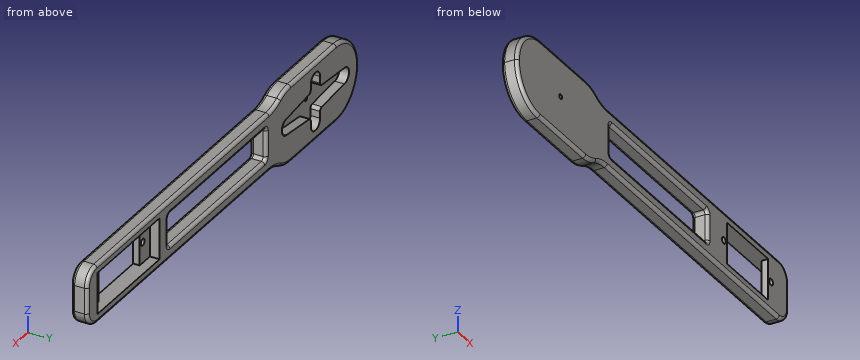
```python
from build123d import *

# Parameters (mm, degrees)
BOSS_EXTRUDE1_DEPTH = 6
CUT_EXTRUDE2_START  = -1
CUT_EXTRUDE2_DEPTH  = 1
SKETCH17_R          = 0.75
CUT_EXTRUDE8_DEPTH  = 4
SKETCH18_R          = 0.75
CUT_EXTRUDE9_DEPTH  = 107.032849905
SKETCH19_W          = 33.2
SKETCH19_H          = 12.8
CUT_EXTRUDE10_DEPTH = 4
SKETCH20_R          = 1
SKETCH20_W          = 22.23131136
SKETCH20_H          = 12.8
CUT_EXTRUDE11_DEPTH = 106.957374727
CUT_EXTRUDE14_DEPTH = 107.084707941
CUT_EXTRUDE15_DEPTH = 101.853925106
FILLET1_R           = 5
CUT_EXTRUDE16_DEPTH = 10
FILLET2_R           = 12
FILLET3_R           = 12
FILLET4_R           = 12
FILLET5_R           = 12
FILLET6_R           = 1
FILLET7_R           = 1


# Read off the part's stored shape, not the designer's step: Cut-Extrude2
# Some blends are built 0.0001 mm under size
with BuildPart() as part:
    # Sketch1 → Boss-Extrude1 (new body)
    with BuildSketch(Plane(origin=(0, 0, 0), x_dir=(1, 0, 0), z_dir=(0, 1, 0))):
        with BuildLine():
            Line((0, 13.97), (47.625, 13.97))
            Line((47.625, 13.97), (47.625, 1.969341724))
            Line((47.625, 1.969341724), (47.625, -12.000658276))
            Line((47.625, -12.000658276), (0, -12.000658276))
            Line((0, -12.000658276), (-47.625, -12.000658276))
            Line((-47.625, -12.000658276), (-50.459972113, -12.000658276))
            ThreePointArc((-50.459972113, -12.000658276), (-102.034450626, 0.984670862), (-50.459972113, 13.97))
            Line((-50.459972113, 13.97), (-47.625, 13.97))
            Line((-47.625, 13.97), (0, 13.97))
        make_face()
    extrude(amount=BOSS_EXTRUDE1_DEPTH)

    # Cut-Extrude2 outline → Cut-Extrude2 (cut)
    with BuildSketch(Plane(origin=(0, 6, 0), x_dir=(1, 0, 0), z_dir=(0, 1, 0)).offset(CUT_EXTRUDE2_START)):
        with BuildLine():
            ThreePointArc((-50.459972113, 13.97), (-102.034450626, 0.984670862), (-50.459972113, -12.000658276))
            Line((-50.459972113, -12.000658276), (47.625, -12.000658276))
            Line((47.625, -12.000658276), (47.625, 13.97))
            Line((47.625, 13.97), (-50.459972113, 13.97))
        make_face()
    extrude(amount=CUT_EXTRUDE2_DEPTH, mode=Mode.SUBTRACT)

    # Sketch17 → Cut-Extrude8 (cut)
    with BuildSketch(Plane(origin=(0, 6, 0), x_dir=(1, 0, 0), z_dir=(0, 1, 0))):
        with BuildLine():
            Line((-59.083269409, 3.484499971), (-71.222931526, 4.833351317))
            ThreePointArc((-71.222931526, 4.833351317), (-71.857628018, 5.160313589), (-72.1125, 5.827235052))
            Line((-72.1125, 5.827235052), (-72.1125, 7.484670862))
            ThreePointArc((-72.1125, 7.484670862), (-74.6125, 9.984670862), (-77.1125, 7.484670862))
            Line((-77.1125, 7.484670862), (-77.1125, 5.377669348))
            ThreePointArc((-77.1125, 5.377669348), (-77.379740938, 4.697181172), (-78.038628314, 4.380401593))
            Line((-78.038628314, 4.380401593), (-90.132022217, 3.484594638))
            ThreePointArc((-90.132022217, 3.484594638), (-92.6125, 0.984670862), (-90.132022217, -1.515252913))
            Line((-90.132022217, -1.515252913), (-78.038628314, -2.411059869))
            ThreePointArc((-78.038628314, -2.411059869), (-77.379740938, -2.727839448), (-77.1125, -3.408327624))
            Line((-77.1125, -3.408327624), (-77.1125, -5.515329138))
            ThreePointArc((-77.1125, -5.515329138), (-74.6125, -8.015329138), (-72.1125, -5.515329138))
            Line((-72.1125, -5.515329138), (-72.1125, -3.857893328))
            ThreePointArc((-72.1125, -3.857893328), (-71.857628018, -3.190971865), (-71.222931526, -2.864009593))
            Line((-71.222931526, -2.864009593), (-59.083269409, -1.515158247))
            ThreePointArc((-59.083269409, -1.515158247), (-56.6125, 0.984670862), (-59.083269409, 3.484499971))
        make_face()
        with Locations(Location((-74.6125, 0.984670862, 0), (0, 0, 270))):
            Circle(SKETCH17_R, mode=Mode.SUBTRACT)
    extrude(amount=-CUT_EXTRUDE8_DEPTH, mode=Mode.SUBTRACT)

    # Sketch18 → Cut-Extrude9 (cut, through all)
    with BuildSketch(Plane(origin=(0, 5, 0), x_dir=(1, 0, 0), z_dir=(0, 1, 0))):
        with Locations(Location((-74.6125, 0.984670862, 0), (0, 0, 270))):
            Circle(SKETCH18_R)
    extrude(amount=-CUT_EXTRUDE9_DEPTH, mode=Mode.SUBTRACT)

    # Sketch19 → Cut-Extrude10 (cut)
    with BuildSketch(Plane(origin=(0, 6, 0), x_dir=(1, 0, 0), z_dir=(0, 1, 0))):
        with Locations((25.585, 0.984670862)):
            Rectangle(SKETCH19_W, SKETCH19_H)
    extrude(amount=-CUT_EXTRUDE10_DEPTH, mode=Mode.SUBTRACT)

    # Sketch20 → Cut-Extrude11 (cut, through all)
    with BuildSketch(Plane(origin=(0, 2, 0), x_dir=(1, 0, 0), z_dir=(0, 1, 0))):
        with Locations(Location((12.885, 0.984670862, 0), (0, 0, 270))):
            Circle(SKETCH20_R)
        with Locations(Location((38.285, 0.984670862, 0), (0, 0, 270))):
            Circle(SKETCH20_R)
        with Locations((25.575892078, 0.984670862)):
            Rectangle(SKETCH20_W, SKETCH20_H)
    extrude(amount=-CUT_EXTRUDE11_DEPTH, mode=Mode.SUBTRACT)

    # Sketch21 → Cut-Extrude14 (cut, through all)
    with BuildSketch(Plane(origin=(0, 6, 0), x_dir=(1, 0, 0), z_dir=(0, 1, 0))):
        with BuildLine():
            Line((-53.303512895, 9.984670862), (47.625, 9.984670862))
            Line((47.625, 9.984670862), (47.625, 13.97))
            Line((47.625, 13.97), (-50.459972113, 13.97))
            ThreePointArc((-50.459972113, 13.97), (-102.034450626, 0.984670862), (-50.459972113, -12.000658276))
            Line((-50.459972113, -12.000658276), (47.625, -12.000658276))
            Line((47.625, -12.000658276), (47.625, -8.015329138))
            Line((47.625, -8.015329138), (-53.303512895, -8.015329138))
            ThreePointArc((-53.303512895, -8.015329138), (-97.74414351, 0.984670862), (-53.303512895, 9.984670862))
        make_face()
    extrude(amount=-CUT_EXTRUDE14_DEPTH, mode=Mode.SUBTRACT)

    # Sketch23 → Cut-Extrude15 (cut, through all)
    with BuildSketch(Plane(origin=(0, 6, 0), x_dir=(1, 0, 0), z_dir=(0, 1, 0))):
        with BuildLine():
            Line((-48.303512895, 4.984670862), (-48.303512895, -3.015329138))
            ThreePointArc((-48.303512895, -3.015329138), (-48.010619676, -3.722435919), (-47.303512895, -4.015329138))
            Line((-47.303512895, -4.015329138), (3.485, -4.015329138))
            ThreePointArc((3.485, -4.015329138), (4.192106781, -3.722435919), (4.485, -3.015329138))
            Line((4.485, -3.015329138), (4.485, 4.984670862))
            ThreePointArc((4.485, 4.984670862), (4.192106781, 5.691777643), (3.485, 5.984670862))
            Line((3.485, 5.984670862), (-47.303512895, 5.984670862))
            ThreePointArc((-47.303512895, 5.984670862), (-48.010619676, 5.691777643), (-48.303512895, 4.984670862))
        make_face()
    extrude(amount=-CUT_EXTRUDE15_DEPTH, mode=Mode.SUBTRACT)

    # Fillet1
    fillet1_edges = [part.edges().sort_by_distance(p)[0] for p in [
        (47.625, 2.5, 8.015329138),
        (47.625, 2.5, -9.984670862),
    ]]
    fillet(fillet1_edges, radius=FILLET1_R)

    # Sketch25 → Cut-Extrude16 (cut)
    with BuildSketch(Plane(origin=(0, 5, 0), x_dir=(1, 0, 0), z_dir=(0, 1, 0))):
        with BuildLine():
            Line((-94.388063999, -11.015329138), (-54.836936001, -11.015329138))
            ThreePointArc((-54.836936001, -11.015329138), (-74.6125, -22.146972648), (-94.388063999, -11.015329138))
        make_face()
        with BuildLine():
            Line((-94.388063999, 12.984670862), (-54.836936001, 12.984670862))
            ThreePointArc((-54.836936001, 12.984670862), (-74.6125, 24.116314372), (-94.388063999, 12.984670862))
        make_face()
    extrude(amount=-CUT_EXTRUDE16_DEPTH, mode=Mode.SUBTRACT)

    # Fillet2
    # the kernel refuses this fillet: 12 mm, written as the material it takes off along each edge
    with BuildSketch(Plane(origin=(-54.836936001, 21.009577066, -12.984670862), x_dir=(-1, 0, 0), z_dir=(0, -1, 0))) as fillet2_piece_1:
        with BuildLine():
            CenterArc((6.403830826, -12), FILLET2_R, 90, 41.409622109)
            Line((-1.533423107, -3), (-1.692168186, -2.82))
            ThreePointArc((-1.692168186, -2.82), (-1.035105589, -1.362812794), (-0.20517934, 0.124504772))
            Line((-0.20517934, 0.124504772), (0, 0.24))
            Line((0, 0.24), (6.403830826, 0.24))
            Line((6.403830826, 0.24), (6.403830826, 0))
        make_face()
    extrude(amount=37.019154131, mode=Mode.SUBTRACT)

    # Fillet3
    fillet3_edges = [part.edges().sort_by_distance(p)[0] for p in [
        (-94.388063999, 2.5, 11.015329138),
        (-94.388063999, 2.5, -12.984670862),
    ]]
    fillet(fillet3_edges, radius=FILLET3_R - 0.0001)  # a hair under: the kernel refuses the full size

    # Fillet4
    # the kernel refuses this fillet: 12 mm, written as the material it takes off along each edge
    with BuildSketch(Plane(origin=(-54.836936001, 21.009577066, 11.015329138), x_dir=(-1, 0, 0), z_dir=(0, -1, 0))) as fillet4_piece_1:
        with BuildLine():
            CenterArc((6.403830826, 12), FILLET4_R, 228.590377891, 41.409622109)
            Line((-1.533423107, 3), (-1.692168186, 2.82))
            ThreePointArc((-1.692168186, 2.82), (-1.035105589, 1.362812794), (-0.20517934, -0.124504772))
            Line((-0.20517934, -0.124504772), (0, -0.24))
            Line((0, -0.24), (6.403830826, -0.24))
            Line((6.403830826, -0.24), (6.403830826, 0))
        make_face()
    extrude(amount=37.019154131, mode=Mode.SUBTRACT)

    # Fillet5
    fillet5_edges = [part.edges().sort_by_distance(p)[0] for p in [
        (-53.303512895, 2.5, -9.984670862),
        (-53.303512895, 2.5, 8.015329138),
    ]]
    fillet(fillet5_edges, radius=FILLET5_R)

    # Fillet6
    fillet6_edges = [part.edges().sort_by_distance(p)[0] for p in [
        (-3.498408395, 5, 8.015329138),
        (-3.498408395, 0, 8.015329138),
        (47.625, 5, -0.984670862),
        (46.160533906, 5, -8.520204768),
        (46.160533906, 5, 6.550863044),
        (47.625, 0, -0.984670862),
        (46.160533906, 0, -8.520204768),
        (46.160533906, 0, 6.550863044),
        (-58.240766828, 0, -12.603620901),
        (-73.492505169, 5, -12.984670862),
        (-94.22941606, 5, -9.470019638),
        (-94.22941606, 5, 7.500677914),
        (-73.492505169, 0, -12.984670862),
        (-94.22941606, 0, -9.470019638),
        (-94.22941606, 0, 7.500677914),
        (-73.492505169, 0, 11.015329138),
        (-73.492505169, 5, 11.015329138),
        (-58.240766828, 5, 10.634279177),
        (-58.240766828, 0, 10.634279177),
        (-3.498408395, 5, -9.984670862),
        (-3.498408395, 0, -9.984670862),
        (-58.240766828, 5, -12.603620901),
        (-52.621816789, 5, 8.396379099),
        (-52.621816789, 0, 8.396379099),
        (-52.621816789, 5, -10.365720823),
        (-52.621816789, 0, -10.365720823),
    ]]
    fillet(fillet6_edges, radius=FILLET6_R)

    # Fillet7
    fillet7_edges = [part.edges().sort_by_distance(p)[0] for p in [
        (-48.303512895, 5, -0.984670862),
        (-48.010619676, 5, 3.722435919),
        (-21.909256447, 5, 4.015329138),
        (4.192106781, 5, 3.722435919),
        (4.485, 5, -0.984670862),
        (4.192106781, 5, -5.691777643),
        (-21.909256447, 5, -5.984670862),
        (-48.010619676, 5, -5.691777643),
        (-48.010619676, 0, -5.691777643),
        (-21.909256447, 0, -5.984670862),
        (4.192106781, 0, -5.691777643),
        (4.485, 0, -0.984670862),
        (4.192106781, 0, 3.722435919),
        (-21.909256447, 0, 4.015329138),
        (-48.010619676, 0, 3.722435919),
        (-48.303512895, 0, -0.984670862),
    ]]
    fillet(fillet7_edges, radius=FILLET7_R)


solid = part.part
```
Input: part model. Units: mm. Frame: model coordinates. Give positions to 0.01 mm unless a question says otherwise; leave off trailing zeros. Order: outer loops, then holes, each group sorted by start corner. A loop starts at its lowest first (then second) coordinate and runs counter-clockwise, first axis right, second up.
1. Material intervals for L1, parallel to X at y = 1, z = -4 (3 decimals); L2, parallel to Z at x = 18, y = 3.7; L3, parallel to Z at x = -8, y = 3.2, sorted ascending.
Derived:
L1: x = -97.359 to -48.304, 4.485 to 14.46, 36.692 to 47.625
L2: z = -9.98 to -7.38, 5.42 to 8.02
L3: z = -9.98 to -5.98, 4.02 to 8.02
2. Pin query (flat end, axial travel): pin 1 (1.8 mm diameter, centred on y = 3, z = -6.5, fed in from -X); pin 2 (1.5 mm diameter, centred on x = 31, y = 3, fed in from +Z); pin 3 (2.5 mm diameter, centred on x = 23.5, y = 1.5, fed in from -Z); pin 4 (6 mm diameter, centred on x = 23, z = -2, fed in from -Y). Return the tip coordinate at first contact, or that it passes through.
Derived:
pin 1: stops at x = -96.82
pin 2: stops at z = 8.02
pin 3: stops at z = -9.98
pin 4: passes through
3. Section A-A on x = 30. Return the cut outline in (y, z), and give its area (3 significant figures).
Derived:
outline: (0, -8.98) arc R1 ccw to (1, -9.98) - (4, -9.98) arc R1 ccw to (5, -8.98) - (5, -7.38) - (0, -7.38) - close; (0, 5.42) - (5, 5.42) - (5, 7.02) arc R1 ccw to (4, 8.02) - (1, 8.02) arc R1 ccw to (0, 7.02) - close
area: 25.1 mm2
4. Section B-B on x = -27.5. Return the cut outline in (y, z), and give its area (3 significant figures).
Derived:
outline: (0, -8.98) arc R1 ccw to (1, -9.98) - (4, -9.98) arc R1 ccw to (5, -8.98) - (5, -6.98) arc R1 ccw to (4, -5.98) - (1, -5.98) arc R1 ccw to (0, -6.98) - close; (0, 5.02) arc R1 ccw to (1, 4.02) - (4, 4.02) arc R1 ccw to (5, 5.02) - (5, 7.02) arc R1 ccw to (4, 8.02) - (1, 8.02) arc R1 ccw to (0, 7.02) - close
area: 38.3 mm2
